Can you work these out from the model? Positions are in its coordinate system, mm. Face numbers are marked on the shaded views. A direction names the side the tool comes from. Coordinates: 2 decimals unless noted, no trailing zeros. Order: outer loops, then holes, each group sorted by start corner. A loop starts at its lowest first (then second) coordinate and runs counter-clockwise, first axis right, second up. Notation, with made-up numbers: M -6.75,0 L 39.25,0 A24 cw 39.25,14 Z; hole C 72,9.5 d9. An arc over 180 degrees is marked long. Answer as a JSON object with one key per item and string values.
from build123d import *

# Parameters (mm, degrees)
SKETCH1_R           = 34.694413408
BOSS_EXTRUDE1_DEPTH = 14.2875
HOLE1_OUTLINE_R     = 6.35
HOLE1_DEPTH         = 5.08
HOLE1_START         = 5.08
HOLE1_2_OUTLINE_R   = 3.175
HOLE1_2_DEPTH       = 9.2075
CHAMFER1_SIZE       = 0.79375
SKETCH9_R           = 3.571875
CUT_EXTRUDE1_DEPTH  = 6.35
SKETCH10_R          = 2.758039836
CUT_EXTRUDE2_DEPTH  = 25.4
CHAMFER2_SIZE       = 0.396875


# Read off the part's stored shape, not the designer's step: Hole1
with BuildPart() as part:
    # Sketch1 → Boss-Extrude1 (new body)
    with BuildSketch(Plane.XY):
        Circle(SKETCH1_R)
    extrude(amount=BOSS_EXTRUDE1_DEPTH)

    # Hole1 outline → Hole1 (cut)
    with BuildSketch(Plane.XY):
        with Locations((21.997045256, -12.7)):
            Circle(HOLE1_OUTLINE_R)
        with Locations((-21.997045256, -12.7)):
            Circle(HOLE1_OUTLINE_R)
        with Locations((0, 25.4)):
            Circle(HOLE1_OUTLINE_R)
    extrude(amount=HOLE1_DEPTH, mode=Mode.SUBTRACT)

    # Hole1 2 outline → Hole1 2 (cut)
    with BuildSketch(Plane.XY.offset(HOLE1_START)):
        with Locations((21.997045256, -12.7)):
            Circle(HOLE1_2_OUTLINE_R)
        with Locations((-21.997045256, -12.7)):
            Circle(HOLE1_2_OUTLINE_R)
        with Locations((0, 25.4)):
            Circle(HOLE1_2_OUTLINE_R)
    extrude(amount=HOLE1_2_DEPTH, mode=Mode.SUBTRACT)

    # Chamfer1
    chamfer1_edges = [part.edges().sort_by_distance(p)[0] for p in [
        (-34.694413408, 0, 0),
        (-34.694413408, 0, 14.2875),
    ]]
    chamfer(chamfer1_edges, length=CHAMFER1_SIZE)

    # Sketch9 → Cut-Extrude1 (cut)
    with BuildSketch(Plane(origin=(0, -34.694413408, 0), x_dir=(-1, 0, 0), z_dir=(0, -1, 0))):
        with Locations(Location((0, -7.14375, 0), (0, 0, 90))):
            Circle(SKETCH9_R)
    extrude(amount=-CUT_EXTRUDE1_DEPTH, mode=Mode.SUBTRACT)

    # Sketch10 → Cut-Extrude2 (cut)
    with BuildSketch(Plane(origin=(0, -28.344413408, 0), x_dir=(-1, 0, 0), z_dir=(0, -1, 0))):
        with Locations(Location((0, -7.14375, 0), (0, 0, 90))):
            Circle(SKETCH10_R)
    extrude(amount=-CUT_EXTRUDE2_DEPTH, mode=Mode.SUBTRACT)

    # Chamfer2
    chamfer2_edges = [part.edges().sort_by_distance(p)[0] for p in [
        (-28.347045256, -12.7, 0),
        (-6.35, 25.4, 0),
        (15.647045256, -12.7, 0),
    ]]
    chamfer(chamfer2_edges, length=CHAMFER2_SIZE)


solid = part.part
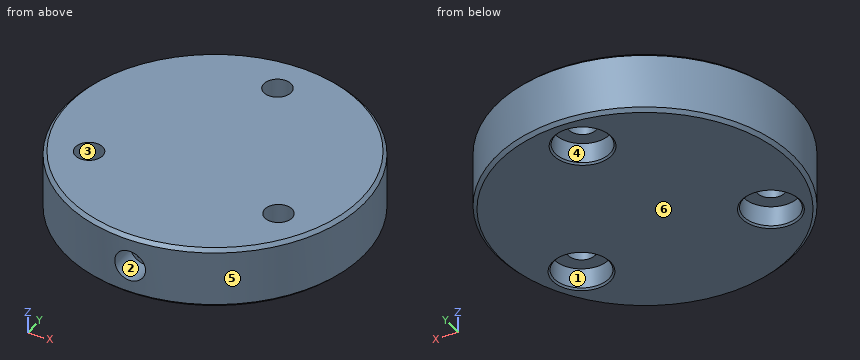
Item 1: I want a section at B-B, the plane z = 6.5. Write out the boundary of the cut face in (x, y) (3 decimals).
Answers follow:
{"outline": "M -3.513,-34.516 L -3.513,-28.344 L -2.682,-28.344 L -2.682,-2.944 L 2.682,-2.944 L 2.682,-28.344 L 3.513,-28.344 L 3.513,-34.516 A34.694 ccw long Z; hole C -21.997,-12.7 d6.35; hole C 0,25.4 d6.35; hole C 21.997,-12.7 d6.35"}
Item 2: Please list where these lines run through material, in increasing order: line 1 (Y direction, x = 0, z = 1.7); line 2 (X direction, y = -13, z = 3.5); line 3 (Y direction, x = 0, z = 11.25) (3 decimals).
Answers follow:
{"line 1": "y = -34.69 to 19.05, 31.75 to 34.69", "line 2": "x = -32.17 to -28.34, -15.65 to 15.65, 28.34 to 32.17", "line 3": "y = -34.694 to 22.225, 28.575 to 34.694"}
Item 3: I'm going to push flat-ended pins straight in: pin 1 (7 mm diameter, centred on x = 0, z = 7.14, fed in from -Y); pin 2 (4.5 mm diameter, centred on x = 1.5, z = 8, fed in from -Y); pin 3 (5.5 mm diameter, centred on x = -22, y = -12.7, fed in from +Z); pin 4 (8 mm diameter, centred on y = -11, z = 12.5, fed in from +X). Where does each tip first touch, or does it pass through?
Answers follow:
{"pin 1": "stops at y = -28.34", "pin 2": "stops at y = -34.65", "pin 3": "passes through", "pin 4": "stops at x = 33.98"}
Item 4: I want a section at D-D, the plane z = 12. Write out the boundary of the cut face in (x, y) (3 decimals).
Answers follow:
{"outline": "C 0,0 d69.389; hole C -21.997,-12.7 d6.35; hole C 0,25.4 d6.35; hole C 21.997,-12.7 d6.35"}
Item 5: I want a section at C-C, the plane y = -12.7. Give the number of separate pieces and of enclosed holes in the cut face, plus the area to 3 significant figures.
Answers follow:
{"separate pieces": "3", "enclosed holes": "1", "area": "651 mm^2"}
Item 6: If we mould it in two halves opening along Y, with no side actions, what happens to the marked faces 4, 5 and 6? For each: pulls with the +Y half, pulls with the -Y half, needs draft (parallel to the pull), parting line crosses it, or undercut.
Answers follow:
{"face 4": "undercut", "face 5": "parting line crosses it", "face 6": "needs draft"}
Item 7: Which directions (+Z, -Z, +X, -X, +Y, -Y) give clear straight access to the entire face, cutting with the end or side of a thin tool? Please do the marked faces 1, 2 and 3.
Answers follow:
{"face 1": "-Z", "face 2": "-Y", "face 3": "+Z, -Z"}
